Can you work these out from the model? Positions are in its coordinate system, mm. Round coordinates to 2 decimals unless told otherwise and drop trailing zeros. Loops run counter-clockwise (first coordinate to the right, second up) from the corner with the lowest first, then second, coordinate; pieces in that order, holes last.
(1) If I drill on line 1 along Y through (x, z) = (-0.5, 193); line 2 along Y through (x, z) = (-0.25, 256.5), over which ranges is the centre line in solid material (lowest first)?
(2) I want a section at B-B on z = 20. Write out the boundary of the cut face in (x, y).
(3) I want a section at A-A on z = 110. Write out the boundary of the cut face in (x, y), plus the area to 3 significant figures.
(4) Will these pins go through, and if not, where does the flat tip stop? pin 1 Ø6 at (x, z) = (1, 253) entering from -Y; pin 2 Ø5 at (x, y) = (2.5, -1) entering from -Z; pin 3 Ø1.5 at (y, z) = (-2, 85.5) entering from +X; pin 4 Ø5 at (y, z) = (-3.5, 122.5) entering from -X.
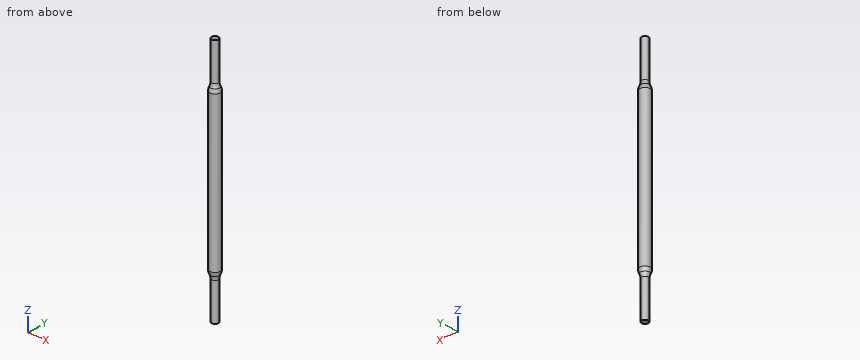
from build123d import *

# Parameters (mm, degrees)
SKETCH1_R           = 4
BOSS_EXTRUDE1_DEPTH = 50
SKETCH2_R           = 6.25
BOSS_EXTRUDE2_DEPTH = 185
SKETCH3_R           = 4
BOSS_EXTRUDE3_DEPTH = 50
FILLET1_R           = 10
FILLET2_R           = 10


with BuildPart() as part:
    # Sketch1 → Boss-Extrude1 (new body)
    with BuildSketch(Plane.XY):
        Circle(SKETCH1_R)
    extrude(amount=BOSS_EXTRUDE1_DEPTH)

    # Sketch2 → Boss-Extrude2 (add)
    with BuildSketch(Plane.XY.offset(50)):
        Circle(SKETCH2_R)
    extrude(amount=BOSS_EXTRUDE2_DEPTH)

    # Sketch3 → Boss-Extrude3 (add)
    with BuildSketch(Plane.XY.offset(235)):
        Circle(SKETCH3_R)
    extrude(amount=BOSS_EXTRUDE3_DEPTH)

    # Fillet1
    # the kernel refuses this fillet: 10 mm, written as the material it adds along each edge
    with BuildSketch(Plane(origin=(0, 0, 235), x_dir=(1, 0, 0), z_dir=(0, -1, 0))) as fillet1_piece_1:
        with BuildLine():
            CenterArc((14, 6.31961233), FILLET1_R, 180, 39.194967426)
            Line((4, 6.31961233), (3.8, 6.31961233))
            Line((3.8, 6.31961233), (3.8, 0))
            Line((3.8, 0), (4, -0.2))
            ThreePointArc((4, -0.2), (5.125, -0.2), (6.095, -0.126392247))
            Line((6.095, -0.126392247), (6.25, 0))
        make_face()
    revolve(axis=Axis((0, 0, 235), (0, 0, 1)))
    with BuildSketch(Plane(origin=(0, 0, 50), x_dir=(1, 0, 0), z_dir=(0, -1, 0))) as fillet1_piece_2:
        with BuildLine():
            CenterArc((14, -6.31961233), FILLET1_R, 140.805032574, 39.194967426)
            Line((4, -6.31961233), (3.8, -6.31961233))
            Line((3.8, -6.31961233), (3.8, 0))
            Line((3.8, 0), (4, 0.2))
            ThreePointArc((4, 0.2), (5.125, 0.2), (6.095, 0.126392247))
            Line((6.095, 0.126392247), (6.25, 0))
        make_face()
    revolve(axis=Axis((0, 0, 50), (0, 0, 1)))

    # Fillet2
    fillet2_edges = [part.edges().sort_by_distance(p)[0] for p in [
        (-6.25, 0, 50),
        (-6.25, 0, 235),
    ]]
    fillet(fillet2_edges, radius=FILLET2_R)


solid = part.part
Filled sheet:
1. line 1: y = -6.23 to 6.23
1. line 2: y = -3.99 to 3.99
2. outline: circle Ø8 at (0, 0)
3. outline: circle Ø12.5 at (0, 0)
3. area: 123 mm2
4. pin 1: stops at y = -4
4. pin 2: stops at z = 0
4. pin 3: stops at x = 6.12
4. pin 4: stops at x = -6.17
